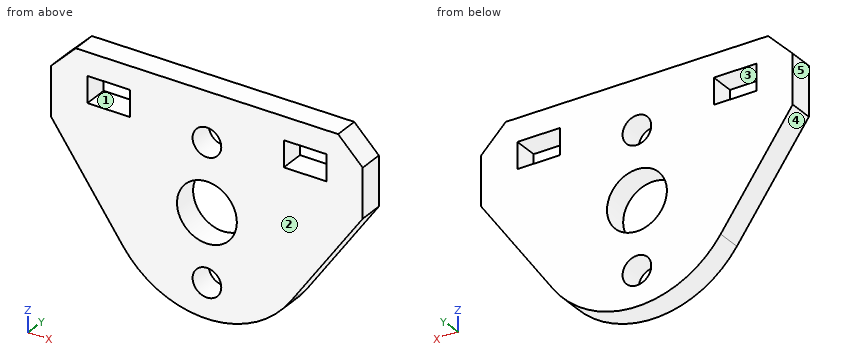
```python
from build123d import *

# Parameters (mm, degrees)
SKETCH003_R             = 3.65
SKETCH003_W             = 5.2
SKETCH003_H             = 3.2
PAD003_DEPTH            = 3
SKETCH009_R             = 1.75
POCKET004_DEPTH         = 3.001
CHAMFER_SIZE            = 3
BODY002_PLACEMENT_ANGLE = 90


with BuildPart() as part:
    # Sketch003 → Pad003 (new body)
    with BuildSketch(Plane.XY):
        with BuildLine():
            Line((-19, 14.267973), (19, 14.267973))
            Line((19, 14.267973), (19, 5.267973))
            Line((19, 5.267973), (10.219447, -7.198118))
            ThreePointArc((-10.219436, -7.198133), (9e-06, -12.5), (10.219447, -7.198118))
            Line((-19, 5.267973), (-10.219436, -7.198133))
            Line((-19, 5.267973), (-19, 14.267973))
        make_face()
        Circle(SKETCH003_R, mode=Mode.SUBTRACT)
        with Locations((-11.975, 9.867973)):
            Rectangle(SKETCH003_W, SKETCH003_H, mode=Mode.SUBTRACT)
        with Locations((11.975, 9.867973)):
            Rectangle(SKETCH003_W, SKETCH003_H, mode=Mode.SUBTRACT)
    extrude(amount=PAD003_DEPTH)

    # Sketch009 (on Face17 of Pad003) → Pocket004 (cut, through all)
    with BuildSketch(Plane.XY.offset(3)):
        with Locations((0, 8.25)):
            Circle(SKETCH009_R)
        with Locations((0, -8.25)):
            Circle(SKETCH009_R)
    extrude(amount=-POCKET004_DEPTH, mode=Mode.SUBTRACT)

    # Chamfer
    chamfer_edges = [part.edges().sort_by_distance(p)[0] for p in [
        (-19, 14.267973, 1.5),
        (19, 14.267973, 1.5),
    ]]
    chamfer(chamfer_edges, length=CHAMFER_SIZE)


with BuildPart() as part_1:
    # Body002 placement: moved
    add(part.part.moved(Location((-67, -82, -8))).rotate(Axis((-67, -82, -8), (1, 0, 0)), BODY002_PLACEMENT_ANGLE))


solid = part_1.part
```
The model under review builds one solid part; all positions refer to its coordinate system, in mm. Face numbers are marked on the shaded views. A direction names the side the tool comes from. Coordinates: 2 decimals unless noted, no trailing zeros. Order: outer loops, then holes, each group sorted by start corner. A loop starts at its lowest first (then second) coordinate and runs counter-clockwise, first axis right, second up. Notation, with made-up numbers: M 28.25,-18 L 69.25,-18 A17 ccw 69.25,8 Z; hole C -14.5,55 d3. An arc over 180 degrees is marked long. One line per question, with ' | ' between items.
(1) Insertion check: pin 1 (1.5 mm diameter, centred on x = -76.5, y = -84, fed in from -Z); pin 2 (2 mm diameter, centred on x = -65.5, z = -6, fed in from +Y). Each pin has a flat end and moves straight along its axis. Give the tip position at first contact, or say it passes through.
Geometry results:
pin 1: stops at z = -16.93 | pin 2: passes through
(2) Add section B-B, the plane z = -17.25. Write out the cut boundary in (x, y), then the cut area to 3 significant figures.
Geometry results:
outline: M -75.41,-85 L -68.44,-85 L -68.44,-82 L -75.41,-82 Z; M -65.56,-85 L -58.59,-85 L -58.59,-82 L -65.56,-82 Z | area: 41.8 mm²
(3) Add section C-C, the plane x = -67. Write out the cut boundary in (y, z).
Geometry results:
outline: M -85,-20.5 L -82,-20.5 L -82,-18 L -85,-18 Z; M -85,-14.5 L -82,-14.5 L -82,-11.65 L -85,-11.65 Z; M -85,-4.35 L -82,-4.35 L -82,-1.5 L -85,-1.5 Z; M -85,2 L -82,2 L -82,6.27 L -85,6.27 Z
(4) The part is to be moulded in two halves that separate along Z. For the marked faces 3, 4 and 5, say which applies: +Z half, -Z half, draft (parallel to the pull), parting line (faces both ways), or undercut.
Geometry results:
face 3: undercut | face 4: -Z half | face 5: draft
(5) Machinability: for the marked faces 1 and 2, which of the approach directions +Z, -Z, +X, -X, +Y, -Y give a long, thin tool a straight path to every point of the face, cutting with its end or side? Answer none if there is none.
Geometry results:
face 1: +Y, -Y | face 2: +Z, -Z, +X, -X, -Y
(6) For probe 1 along Z at (x, y) = (-67, -83.65); probe 2 along X at (y, z) = (-83.3, 1.5) (3 decimals); probe 3 along X at (y, z) = (-82.6, 0.5) (3 decimals), list the stretches that pass through material, from the lowest coordinate up. Write a range as from..to.
Geometry results:
probe 1: z = -20.5..-18, -14.5..-11.65, -4.35..-1.5, 2..6.27 | probe 2: x = -86..-81.575, -76.375..-68.225, -65.775..-57.625, -52.425..-48 | probe 3: x = -86..-81.575, -76.375..-68.732, -65.268..-57.625, -52.425..-48
(7) Add section D-D, the plane z = 1. Write out the cut boundary in (x, y) (3 decimals).
Geometry results:
outline: M -86,-85 L -81.575,-85 L -81.575,-82 L -86,-82 Z; M -76.375,-85 L -68.581,-85 L -68.581,-82 L -76.375,-82 Z; M -65.419,-85 L -57.625,-85 L -57.625,-82 L -65.419,-82 Z; M -52.425,-85 L -48,-85 L -48,-82 L -52.425,-82 Z
(8) Add section A-A, the plane y = -82.5. Write out the cut boundary in (x, z) (3 decimals), then the cut area to 3 significant figures.
Geometry results:
outline: M -86,-2.732 L -77.219,-15.198 A12.5 ccw -56.781,-15.198 L -48,-2.732 L -48,3.268 L -51,6.268 L -83,6.268 L -86,3.268 Z; hole M -81.575,0.268 L -76.375,0.268 L -76.375,3.468 L -81.575,3.468 Z; hole C -67,-8 d7.3; hole C -67,-16.25 d3.5; hole C -67,0.25 d3.5; hole M -57.625,0.268 L -52.425,0.268 L -52.425,3.468 L -57.625,3.468 Z | area: 679 mm²
